The listing builds one solid part. Answer for the finished solid, in the listing's coordinates (mm). A direction names the side the tool comes from. Coordinates: 2 decimals unless noted, no trailing zeros. Write each loop counter-clockwise with the first axis right and the second up, starting at its lowest first coordinate (ties: lowest second). Pieces come first, ordered by that corner, then holes. Notation, with made-up numbers: M 48.25,28.25 L 102.25,28.25 A7 cw 102.25,38.25 Z; hole C 74.25,51.25 d3. An arc over 180 degrees is marked long. Answer as CSV lines item,"result".
```python
from build123d import *

# Parameters (mm, degrees)
F0_R     = 3
F1_DEPTH = 11
F3_DEPTH = 2
F2_R     = 17.5
F4_DEPTH = 4
F5_R     = 1.9313708499
F7_R     = 2
F8_DEPTH = 6.5


# Not quite as in the source:
# - a fillet or chamfer that OpenCascade refuses, or shapes differently, is made with other operations: its cross-section is extruded or revolved along the edge and cut away or added


with BuildPart() as f1:
    # F0 (on Front) → F1 (new body)
    with BuildSketch(Plane.XZ):
        Circle(F0_R)
    extrude(amount=-F1_DEPTH)

    # F0 (on Front) → F3 (join)
    with BuildSketch(Plane.XZ):
        Circle(F0_R)
    extrude(amount=F3_DEPTH)

    # F2 (on Front) → F4 (join)
    with BuildSketch(Plane.XZ):
        Circle(F2_R)
    extrude(amount=-F4_DEPTH)

    # F5
    f5_edges = [f1.edges().sort_by_distance(p)[0] for p in [
        (-17.5, 0, 0),
    ]]
    fillet(f5_edges, radius=F5_R)

    # F6: fillet of radius 2.4142135624 on 1 edges, made by hand

    # F6_s1 → F6_t2 (revolve, cut)
    with BuildSketch(Plane.XY):
        with BuildLine():
            ThreePointArc((17.5, 1.9313708499), (16.6908565976, 3.4109907686), (15.1106489294, 4))
            Line((15.1106489294, 4), (15.1106489294, 4.0482842712))
            Line((15.1106489294, 4.0482842712), (17.5, 4.0482842712))
            Line((17.5, 4.0482842712), (17.5482842712, 4))
            ThreePointArc((17.5482842712, 4), (17.5482842712, 2.9656854249), (17.5477870214, 1.9382825381))
            Line((17.5477870214, 1.9382825381), (17.5, 1.9313708499))
        make_face()
    revolve(axis=Axis((0, 4, 0), (0, -1, 0)), mode=Mode.SUBTRACT)

    # F7 (on face) → F8 (cut)
    with BuildSketch(Plane.XZ):
        with Locations((0, -5.9548519258)):
            Circle(F7_R)
        with Locations((6.2130242586, 0)):
            Circle(F7_R)
        with Locations((4.9334257519, 4.926879719)):
            Circle(F7_R)
        with Locations((0, 7)):
            Circle(F7_R)
        with Locations((4.6638702957, -4.2616006167)):
            Circle(F7_R)
        with Locations((-4.2754073071, -3.8503200899)):
            Circle(F7_R)
        with Locations((-4.2925996605, 4.681295439)):
            Circle(F7_R)
        with Locations((-5.8032550169, 0.1451130412)):
            Circle(F7_R)
    extrude(amount=-F8_DEPTH, mode=Mode.SUBTRACT)


solid = f1.part
```
Q1. For faces 4 (the cylindrical face through (-3, 7, 0)), 5 (the cylindrical face through (6.84, 1.97, 5.53)), determine the directions among +Z, -Z, +X, -X, +Y, -Y from which every point of the face is accessible in a straight line to the end or side of a thin tool.
Output:
face 4,"+Y"
face 5,"+Y, -Y"
Q2. Find section C-C (y = 8.5). Give the vertices of the cut face in (x, z).
Output:
outline,"C 0,0 d6"
Q3. Flat-ended cylindrical pins translate along their axes: pin 1 Ø2.5 at (x, z) = (4.93, 4.93) entering from +Y; pin 2 Ø6.5 at (x, z) = (-4.29, 4.68) entering from +Y; pin 3 Ø10 at (x, z) = (-6, 12) entering from -Y; pin 4 Ø4 at (y, z) = (-0.5, -6) entering from +X. Find the tip coordinate at first contact, or state that the pin passes through.
Output:
pin 1,"through"
pin 2,"y = 4"
pin 3,"y = 0"
pin 4,"x = 16.64"
Q4. Find section B-B (z = 4). Count the separate pieces of the cut face and the enclosed holes in it, and give its area (3 significant figures).
Output:
separate pieces,"3"
enclosed holes,"0"
area,"103 mm2"
Q5. Find section A-A (x = 0). Give the vertices of the cut face in (y, z).
Output:
outline,"M -2,-3 L 0,-3 L 0,-3.95 L 4,-3.95 L 4,-3 L 11,-3 L 11,3 L 4,3 L 4,5 L 0,5 L 0,3 L -2,3 Z; M 0,-15.57 A1.93 ccw 1.93,-17.5 A2.41 ccw 4,-15.11 L 4,-7.95 L 0,-7.95 Z; M 0,9 L 4,9 L 4,15.11 A2.41 ccw 1.93,17.5 A1.93 ccw 0,15.57 Z"
Q6. Straight lines are drawn through the part: line 1 (X direction, y = 3.5, z = 4.5); line 2 (Z direction, x = -0.5, y = 3.75); line 3 (Z direction, x = 4, y = 1.5) (3 decimals). For each, find the intervals that lie inside material, in ascending order.
Output:
line 1,"-15.96 to -6.28, -2.3 to 2.98, 6.89 to 15.96"
line 2,"-16.17 to -7.89, -4.02 to 5.06, 8.94 to 16.17"
line 3,"-16.987 to -6.148, -2.375 to 3.158, 6.696 to 16.987"
Q7. The mould has two halves that part along X. Classify faces 1 (the cylindrical face through (0, 2, 9)), 2 (the cylindrical face through (-3, -1, 0)), 3 (the flat face through (3.15, 4, 0.21)): pulls with the +X half, pulls with the -X half, needs draft (parallel to the pull), parting line crosses it, or undercut.
Output:
face 1,"undercut"
face 2,"parting line crosses it"
face 3,"needs draft"
